Geometry check sheet. Reference: the model listing, model coordinates, mm. A direction names the side the tool comes from. Round coordinates to 2 decimals unless told otherwise and drop trailing zeros. Order: outer loops, then holes, each group sorted by start corner. A loop starts at its lowest first (then second) coordinate and runs counter-clockwise, first axis right, second up. Notation, with made-up numbers: (78, -0.5) - (91, -0.5) arc R27 cw to (91, 32.5) - close; hole circle Ø6 at (22.25, 48). An arc over 180 degrees is marked (long way). Return JSON: item names as keys, results as strings. Group by question number.
Q1. Draft check along Z on faces 5 (the cylindrical face through (20.4, -17.44, 72.62)), 6 (the flat face through (13.5, -18, 69)), 7 (the flat face through (0, 21, 28.25)). Enter one of: pulls with the +Z half, pulls with the -Z half, needs draft (parallel to the pull), parting line crosses it, or undercut.
Q2. Sectioned sample at B-B, the plane z = 47.5. Record the cut outline in (x, y).
Q3. Sectioned sample at D-D, the plane y = -17.5. Give the number of separate pieces and of enclosed holes in the cut face, then the cut area to 3 significant figures.
Q4. Tool access check on faces 1 (the flat face through (3.5, -18, 69)), 2 (the flat face through (-13.5, -18, 69)), 3 (the flat face through (21, 15.5, 72)), 4 (the flat face through (21.8, 15.7, 69.5)). Record the directions out of +Z, -Z, +X, -X, +Y, -Y that give a thin tool (end or side, any length) a straight path to the whole face; none if there is none.
Q5. Gauge pin test, flat ends, axial feed: pin 1 Ø2.5 at (y, z) = (-17.5, 56.5) entering from +X; pin 2 Ø12 at (y, z) = (7, 64) entering from -X; pin 3 Ø3 at (x, y) = (11.5, -9.5) entering from +Z; pin 4 Ø12 at (x, y) = (-3, 1) entering from -Z. Record the tip position at first contact, or that the pin passes through.
Q6. Material ranges on line 1 along Y through (x, z) = (21.8, 72); line 2 along X through (y, z) = (-17.5, 73); line 3 along X through (y, z) = (-11, 57.5), recorded low to high.
Q7. Sectioned sample at A-A, the plane x = 21.8. Record the cut outline in (y, z).
Q8. Sectioned sample at C-C, the plane z = 30. Record the cut outline in (x, y), then the cut area to 3 significant figures.
```python
from build123d import *

# Parameters (mm, degrees)
CROQUIS1_W               = 39
CROQUIS1_H               = 39
SALIENTE_EXTRUIR2_DEPTH  = 75.5
CROQUIS2_W               = 33
CROQUIS2_H               = 33
CORTAR_EXTRUIR1_DEPTH    = 80
CROQUIS11_W              = 33
CROQUIS11_H              = 33
SALIENTE_EXTRUIR3_DEPTH  = 37
CROQUIS13_W              = 33
CROQUIS13_H              = 33
CORTAR_EXTRUIR6_DEPTH    = 81.378790735
CROQUIS16_W              = 39
CROQUIS16_H              = 39
CORTAR_EXTRUIR8_DEPTH    = 10
CROQUIS19_W              = 20
CROQUIS19_H              = 20
SALIENTE_EXTRUIR4_DEPTH  = 3
CROQUIS33_W              = 39
CROQUIS33_H              = 39
SALIENTE_EXTRUIR7_DEPTH  = 18
CROQUIS35_W              = 39
CROQUIS35_H              = 39
CORTAR_EXTRUIR17_DEPTH   = 16
CROQUIS36_R              = 6.75
CORTAR_EXTRUIR18_DEPTH   = 2
CORTAR_EXTRUIR19_REACH   = 89.187
SALIENTE_EXTRUIR10_START = 2
CROQUIS38_W              = 45
CROQUIS38_H              = 45
SALIENTE_EXTRUIR10_DEPTH = 2
CROQUIS39_W              = 7.3
CROQUIS39_H              = 4
SALIENTE_EXTRUIR12_DEPTH = 8
RESPIRADERO1_START       = 31
RESPIRADERO1_OUTLINE_W   = 6
RESPIRADERO1_OUTLINE_H   = 3
RESPIRADERO1_OUTLINE_W_2 = 10
RESPIRADERO1_DEPTH       = 39.5
CHAFL_N7_SIZE            = 3
CROQUIS40_R              = 1.4
CORTAR_EXTRUIR20_DEPTH   = 10
CHAFL_N8_SIZE            = 4
CORTAR_EXTRUIR21_REACH   = 60.983
CROQUIS43_R              = 1.5


# Read off the part's stored shape, not the designer's step: Respiradero1
# Some blends are built 0.0001 mm under size
with BuildPart() as part:
    # Croquis1 → Saliente-Extruir2 (new body)
    with BuildSketch(Plane.XY):
        Rectangle(CROQUIS1_W, CROQUIS1_H)
    extrude(amount=SALIENTE_EXTRUIR2_DEPTH)

    # Croquis2 → Cortar-Extruir1 (cut)
    with BuildSketch(Plane.XY.offset(75.5)):
        Rectangle(CROQUIS2_W, CROQUIS2_H)
    extrude(amount=-CORTAR_EXTRUIR1_DEPTH, mode=Mode.SUBTRACT)

    # Croquis11 → Saliente-Extruir3 (add)
    with BuildSketch(Plane(origin=(0, 0, 0), x_dir=(-1, 0, 0), z_dir=(0, 0, -1))):
        Rectangle(CROQUIS11_W, CROQUIS11_H)
    extrude(amount=-SALIENTE_EXTRUIR3_DEPTH)

    # Croquis13 → Cortar-Extruir6 (cut, through all)
    with BuildSketch(Plane(origin=(0, 0, 0), x_dir=(-1, 0, 0), z_dir=(0, 0, -1))):
        Rectangle(CROQUIS13_W, CROQUIS13_H)
    extrude(amount=-CORTAR_EXTRUIR6_DEPTH, mode=Mode.SUBTRACT)

    # Croquis16 → Cortar-Extruir8 (cut)
    with BuildSketch(Plane(origin=(0, 0, 0), x_dir=(-1, 0, 0), z_dir=(0, 0, -1))):
        Rectangle(CROQUIS16_W, CROQUIS16_H)
    extrude(amount=-CORTAR_EXTRUIR8_DEPTH, mode=Mode.SUBTRACT)

    # Croquis19 → Saliente-Extruir4 (add)
    with BuildSketch(Plane(origin=(0, 19.5, 0), x_dir=(1, 0, 0), z_dir=(0, 1, 0))):
        with Locations((-2, -55.5)):
            Rectangle(CROQUIS19_W, CROQUIS19_H)
    extrude(amount=-SALIENTE_EXTRUIR4_DEPTH)

    # Croquis33 → Saliente-Extruir7 (add)
    with BuildSketch(Plane(origin=(0, 0, 10), x_dir=(-1, 0, 0), z_dir=(0, 0, -1))):
        Rectangle(CROQUIS33_W, CROQUIS33_H)
    extrude(amount=-SALIENTE_EXTRUIR7_DEPTH)

    # Croquis35 → Cortar-Extruir17 (cut)
    with BuildSketch(Plane(origin=(0, 0, 10), x_dir=(-1, 0, 0), z_dir=(0, 0, -1))):
        Rectangle(CROQUIS35_W, CROQUIS35_H)
    extrude(amount=-CORTAR_EXTRUIR17_DEPTH, mode=Mode.SUBTRACT)

    # Croquis36 → Cortar-Extruir18 (cut)
    with BuildSketch(Plane(origin=(0, 0, 26), x_dir=(-1, 0, 0), z_dir=(0, 0, -1))):
        Circle(CROQUIS36_R)
    extrude(amount=-CORTAR_EXTRUIR18_DEPTH, mode=Mode.SUBTRACT)

    # Croquis37 → Cortar-Extruir19 (cut, up to next)
    with BuildSketch(Plane(origin=(0, 19.5, 0), x_dir=(1, 0, 0), z_dir=(0, 1, 0)), mode=Mode.PRIVATE) as cortar_extruir19_sk1:
        with BuildLine():
            ThreePointArc((-5.8e-08, -30.95), (-6.484436966, -32.041924812), (-12.253670087, -35.19726489))
            Line((-12.253670087, -35.19726489), (12.253670087, -66.30273511))
            ThreePointArc((12.253670087, -66.30273511), (14.560271631, -64.167842228), (16.5, -61.694861808))
            Line((16.5, -61.694861808), (16.5, -39.805138192))
            ThreePointArc((16.5, -39.805138192), (9.363005266, -33.303678543), (-5.8e-08, -30.95))
        make_face()
    cortar_extruir19_tool1 = extrude(cortar_extruir19_sk1.sketch, amount=-CORTAR_EXTRUIR19_REACH, mode=Mode.PRIVATE) & part.part
    # Croquis37 → Cortar-Extruir19 (cut, up to next)
    with BuildSketch(Plane(origin=(0, 19.5, 0), x_dir=(1, 0, 0), z_dir=(0, 1, 0)), mode=Mode.PRIVATE) as cortar_extruir19_sk2:
        with BuildLine():
            Line((12.253670087, -66.30273511), (-12.253670087, -35.19726489))
            ThreePointArc((-12.253670087, -35.19726489), (-14.560271631, -37.332157772), (-16.5, -39.805138192))
            Line((-16.5, -39.805138192), (-16.5, -61.694861808))
            ThreePointArc((-16.5, -61.694861808), (-9.363005292, -68.196321443), (0, -70.55))
            ThreePointArc((0, -70.55), (6.484436939, -69.458075197), (12.253670087, -66.30273511))
        make_face()
    cortar_extruir19_tool2 = extrude(cortar_extruir19_sk2.sketch, amount=-CORTAR_EXTRUIR19_REACH, mode=Mode.PRIVATE) & part.part
    add(cortar_extruir19_tool1.solids().sort_by_distance((5.629579, 19.5, 45.099579))[0], mode=Mode.SUBTRACT)
    add(cortar_extruir19_tool2.solids().sort_by_distance((-5.629579, 19.5, 56.400421))[0], mode=Mode.SUBTRACT)

    # Croquis38 → Saliente-Extruir10 (add)
    with BuildSketch(Plane(origin=(0, 19.5, 0), x_dir=(1, 0, 0), z_dir=(0, 1, 0)).offset(SALIENTE_EXTRUIR10_START)):
        with Locations((0, -50.75)):
            Rectangle(CROQUIS38_W, CROQUIS38_H)
        with BuildLine():
            Line((-16.5, -39.805138192), (-16.5, -61.694861808))
            ThreePointArc((-16.5, -61.694861808), (0, -70.55), (16.5, -61.694861808))
            Line((16.5, -61.694861808), (16.5, -39.805138192))
            ThreePointArc((16.5, -39.805138192), (0, -30.95), (-16.5, -39.805138192))
        make_face(mode=Mode.SUBTRACT)
    extrude(amount=-SALIENTE_EXTRUIR10_DEPTH)

    # Croquis39 → Saliente-Extruir12 (add)
    with BuildSketch(Plane.XY.offset(75.5)):
        Polygon((-16.5, 16.5), (-16.5, 19.5), (-23.8, 19.5), (-23.8, 15.5), (-16.5, 15.5), align=None)
        with Locations((-20.15, -17.5)):
            Rectangle(CROQUIS39_W, CROQUIS39_H)
        with Locations((20.15, -17.5)):
            Rectangle(CROQUIS39_W, CROQUIS39_H)
        with Locations((20.15, 17.5)):
            Rectangle(CROQUIS39_W, CROQUIS39_H)
    extrude(amount=-SALIENTE_EXTRUIR12_DEPTH)

    # Respiradero1 outline → Respiradero1 (cut)
    with BuildSketch(Plane.XY.offset(RESPIRADERO1_START)):
        with Locations((-12, -18)):
            Rectangle(RESPIRADERO1_OUTLINE_W, RESPIRADERO1_OUTLINE_H)
        with Locations((0, -18)):
            Rectangle(RESPIRADERO1_OUTLINE_W_2, RESPIRADERO1_OUTLINE_H)
        with Locations((12, -18)):
            Rectangle(RESPIRADERO1_OUTLINE_W, RESPIRADERO1_OUTLINE_H)
    extrude(amount=RESPIRADERO1_DEPTH, mode=Mode.SUBTRACT)

    # Chaflán7
    chafl_n7_edges = [part.edges().sort_by_distance(p)[0] for p in [
        (15, -18, 70.5),
        (-15, -18, 70.5),
        (-15, -18, 31),
        (15, -18, 31),
        (5, -18, 31),
        (5, -18, 70.5),
        (9, -18, 70.5),
        (9, -18, 31),
        (-5, -18, 70.5),
        (-5, -18, 31),
        (-9, -18, 31),
        (-9, -18, 70.5),
    ]]
    chamfer(chafl_n7_edges, length=CHAFL_N7_SIZE - 0.0001)  # a hair under: the kernel refuses the full size

    # Croquis40 → Cortar-Extruir20 (cut)
    with BuildSketch(Plane.XY.offset(75.5)):
        with Locations((-21.8, 17.5)):
            Circle(CROQUIS40_R)
        with Locations((21.8, 17.5)):
            Circle(CROQUIS40_R)
        with Locations((21.8, -17.5)):
            Circle(CROQUIS40_R)
        with Locations((-21.8, -17.5)):
            Circle(CROQUIS40_R)
    extrude(amount=-CORTAR_EXTRUIR20_DEPTH, mode=Mode.SUBTRACT)

    # Chaflán8
    # the kernel refuses this chamfer: 4 mm, written as the material it takes off along each edge
    with BuildSketch(Plane(origin=(-23.8, 19.5, 67.5), x_dir=(-0.02749587661058651, 0, 0.9996219169112968), z_dir=(0, -1, 0)), Plane(origin=(23.8, 5.213268048, 67.5), x_dir=(0.02749587661058651, 0, 0.9996219169112968), z_dir=(0, 1, 0))) as chafl_n8_piece_1:
        Polygon((CHAFL_N8_SIZE * 0.999621916911, -CHAFL_N8_SIZE * 0.0274958766106), (-CHAFL_N8_SIZE * 0.0274958766106, -CHAFL_N8_SIZE * 0.999621916911), (0, 0), align=None)
    extrude(amount=14.286731952, mode=Mode.SUBTRACT)
    with BuildSketch(Plane(origin=(-23.8, -29.786731952, 67.5), x_dir=(-0.02749587661058651, 0, 0.9996219169112968), z_dir=(0, 1, 0))) as chafl_n8_piece_2:
        Polygon((CHAFL_N8_SIZE * 0.999621916911, CHAFL_N8_SIZE * 0.0274958766106), (-CHAFL_N8_SIZE * 0.0274958766106, CHAFL_N8_SIZE * 0.999621916911), (0, 0), align=None)
    extrude(amount=24.573463904, mode=Mode.SUBTRACT)
    with BuildSketch(Plane(origin=(23.8, -29.786731952, 67.5), x_dir=(0.02749587661058651, 0, 0.9996219169112968), z_dir=(0, 1, 0))) as chafl_n8_piece_3:
        Polygon((CHAFL_N8_SIZE * 0.999621916911, -CHAFL_N8_SIZE * 0.0274958766106), (-CHAFL_N8_SIZE * 0.0274958766106, -CHAFL_N8_SIZE * 0.999621916911), (0, 0), align=None)
    extrude(amount=24.573463904, mode=Mode.SUBTRACT)

    # Croquis43 → Cortar-Extruir21 (cut, up to next)
    with BuildSketch(Plane(origin=(0, 0, 26), x_dir=(-1, 0, 0), z_dir=(0, 0, -1)), mode=Mode.PRIVATE) as cortar_extruir21_sk1:
        with Locations((10, -10)):
            Circle(CROQUIS43_R)
    cortar_extruir21_tool1 = extrude(cortar_extruir21_sk1.sketch, amount=-CORTAR_EXTRUIR21_REACH, mode=Mode.PRIVATE) & part.part
    add(cortar_extruir21_tool1.solids().sort_by_distance((-10, -10, 26))[0], mode=Mode.SUBTRACT)


solid = part.part
```
Reply:
{
 "1": {"face 5": "needs draft", "face 6": "undercut", "face 7": "pulls with the -Z half"},
 "2": {"outline": "(-22.5, 19.5) - (-19.5, 19.5) - (-19.5, -19.5) - (-15, -19.5) - (-15, -16.5) - (-16.5, -16.5) - (-16.5, 21.5) - (-22.5, 21.5) - close; (-9, -19.5) - (-5, -19.5) - (-5, -16.5) - (-9, -16.5) - close; (5, -19.5) - (9, -19.5) - (9, -16.5) - (5, -16.5) - close; (15, -19.5) - (19.5, -19.5) - (19.5, 19.5) - (22.5, 19.5) - (22.5, 21.5) - (16.5, 21.5) - (16.5, -16.5) - (15, -16.5) - close"},
 "3": {"separate pieces": "3", "enclosed holes": "3", "area": "1,130 mm^2"},
 "4": {"face 1": "+Y, -Y", "face 2": "-Y", "face 3": "+Z, -Z, +X", "face 4": "-Z, +X, -Y"},
 "5": {"pin 1": "x = 19.5", "pin 2": "x = -19.5", "pin 3": "z = 28", "pin 4": "z = 26"},
 "6": {"line 1": "-19.5 to -18.9, -16.1 to -15.5, 15.5 to 16.1, 18.9 to 21.5", "line 2": "-23.8 to -23.2, -20.4 to 20.4, 23.2 to 23.8", "line 3": "-19.5 to -16.5, 16.5 to 19.5"},
 "7": {"outline": "(-19.5, 69.5) - (-18.9, 69.5) - (-18.9, 75.5) - (-19.5, 75.5) - close; (-16.1, 69.5) - (-15.5, 69.5) - (-15.5, 75.5) - (-16.1, 75.5) - close; (15.5, 69.5) - (16.1, 69.5) - (16.1, 75.5) - (15.5, 75.5) - close; (18.9, 69.5) - (19.5, 69.5) - (19.5, 28.25) - (21.5, 28.25) - (21.5, 73.25) - (19.5, 73.25) - (19.5, 75.5) - (18.9, 75.5) - close"},
 "8": {"outline": "(-22.5, 19.5) - (-19.5, 19.5) - (-19.5, -19.5) - (19.5, -19.5) - (19.5, 19.5) - (22.5, 19.5) - (22.5, 21.5) - (-22.5, 21.5) - close; hole (-16.5, -16.5) - (16.5, -16.5) - (16.5, 16.5) - (-16.5, 16.5) - close", "area": "522 mm^2"}
}
